from build123d import *

# Parameters (mm, degrees)
F0_R        = 16.7132
F1_DEPTH    = 5.08
F2_T1_DEPTH = 172.212
F3_R        = 22.86
F4_R        = 22.86


# Not quite as in the source:
# - a fillet or chamfer that OpenCascade refuses, or shapes differently, is made with other operations: its cross-section is extruded or revolved along the edge and cut away or added


with BuildPart() as f1:
    # F0 (on Front) → F1 (new body)
    with BuildSketch(Plane.XZ):
        Polygon((-91.9353, -25.4), (91.9353, -25.4), (91.9353, 25.4), (28.067, 25.4), (28.067, 16.4), (-28.067, 16.4), (-28.067, 25.4), (-91.9353, 25.4), align=None)
        with Locations((-62.5221, 0)):
            Circle(F0_R, mode=Mode.SUBTRACT)
        with Locations((62.5221, 0)):
            Circle(F0_R, mode=Mode.SUBTRACT)
    extrude(amount=F1_DEPTH)

    # F2: fillet of radius 33.4264 on 4 edges, made by hand

    # F2_s2 → F2_t1 (cut)
    with BuildSketch(Plane.XZ.offset(-83.566)):
        with BuildLine():
            ThreePointArc((91.9353, -8.0264), (82.1449341107, 15.6096341107), (58.5089, 25.4))
            Line((58.5089, 25.4), (91.9353, 25.4))
            Line((91.9353, 25.4), (91.9353, -8.0264))
        make_face()
        with BuildLine():
            ThreePointArc((58.5089, -25.4), (82.1449341107, -15.6096341107), (91.9353, 8.0264))
            Line((91.9353, 8.0264), (91.9353, -25.4))
            Line((91.9353, -25.4), (58.5089, -25.4))
        make_face()
        with BuildLine():
            ThreePointArc((-58.5089, 25.4), (-82.1449341107, 15.6096341107), (-91.9353, -8.0264))
            Line((-91.9353, -8.0264), (-91.9353, 25.4))
            Line((-91.9353, 25.4), (-58.5089, 25.4))
        make_face()
        with BuildLine():
            ThreePointArc((-91.9353, 8.0264), (-82.1449341107, -15.6096341107), (-58.5089, -25.4))
            Line((-58.5089, -25.4), (-91.9353, -25.4))
            Line((-91.9353, -25.4), (-91.9353, 8.0264))
        make_face()
    extrude(amount=F2_T1_DEPTH, mode=Mode.SUBTRACT)

    # F3
    f3_edges = [f1.edges().sort_by_distance(p)[0] for p in [
        (-90.957338, -2.54, 0),
    ]]
    fillet(f3_edges, radius=F3_R)

    # F4
    f4_edges = [f1.edges().sort_by_distance(p)[0] for p in [
        (90.957338, -2.54, 0),
    ]]
    fillet(f4_edges, radius=F4_R)


solid = f1.part
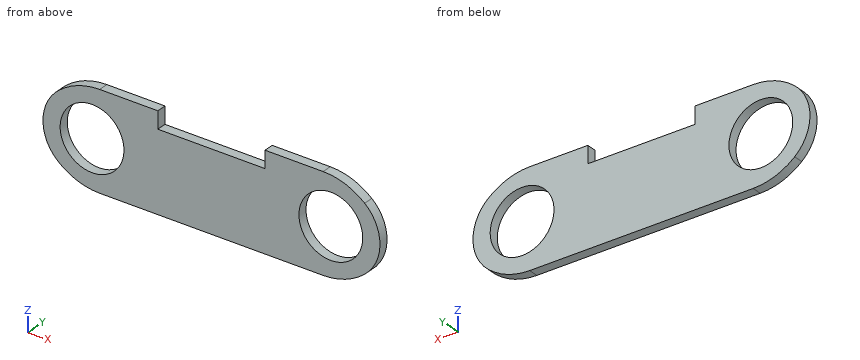
Build history of the part. All positions in model axes, mm. Round coordinates to 2 decimals unless told otherwise and drop trailing zeros. Loops run counter-clockwise (first coordinate to the right, second up) from the corner with the lowest first, then second, coordinate; pieces in that order, holes last. Notation, with made-up numbers: (4.25, 69.25) -> (62.25, 69.25) arc R34 ccw to (62.25, 105.25) -> close; hole circle Ø5 at (68, 88.5). An arc over 180 degrees is marked (long way). Answer in a Markdown table with one row per item.
Item 1: Pin check, flat tips, straight feed: pin 1 (1.5 mm diameter, centred on y = -4, z = 20, fed in from -X); pin 2 (1 mm diameter, centred on y = -3, z = -19.5, fed in from +X); pin 3 (2.5 mm diameter, centred on y = -3, z = 22.5, fed in from +X). Stop position of each tip, or through.
Answers below:
| item | result |
|---|---|
| pin 1 | stops at x = -77.83 |
| pin 2 | stops at x = 78.18 |
| pin 3 | stops at x = 74.64 |
Item 2: Drill centre lines: L1, parallel to X at y = -0.5, z = -8; L2, parallel to X at y = -3.95, z = 4; L3, parallel to Z at x = -12, y = -1.05. Where is each one in solid material? Low to high. Write a range as [from, to].
Answers below:
| item | result |
|---|---|
| L1 | x = [-86.8, -77.2], [-47.85, 47.85], [77.2, 86.8] |
| L2 | x = [-87.89, -78.75], [-46.29, 46.29], [78.75, 87.89] |
| L3 | z = [-25.4, 16.4] |
Item 3: Saw through at B-B (y = -2.15). State how many separate pieces and enclosed holes the cut face has, and give its area (3 significant figures).
Answers below:
| item | result |
|---|---|
| separate pieces | 1 |
| enclosed holes | 2 |
| area | 6,060 mm² |
Item 4: Saw through at A-A (x = -53.5). Write the cut outline in (y, z), and give its area (3 significant figures).
Answers below:
| item | result |
|---|---|
| outline | (-5.08, -25.4) -> (0, -25.4) -> (0, -14.07) -> (-5.08, -14.07) -> close; (-5.08, 14.07) -> (0, 14.07) -> (0, 25.4) -> (-5.08, 25.4) -> close |
| area | 115 mm² |
Item 5: Saw through at D-D (x = 72). Write the cut outline in (y, z), and give its area (3 significant figures).
Answers below:
| item | result |
|---|---|
| outline | (-5.08, -22.56) -> (0, -22.56) -> (0, -13.77) -> (-5.08, -13.77) -> close; (-5.08, 13.77) -> (0, 13.77) -> (0, 22.56) -> (-5.08, 22.56) -> close |
| area | 89.3 mm² |
